from build123d import *

# Parameters (mm, degrees)
F0_W     = 152.4
F0_H     = 1524
F0_W_2   = 114.3
F0_H_2   = 1485.9
F1_DEPTH = 2133.6
F2_W     = 114.3
F2_H     = 19.05
F3_DEPTH = 1485.9
F5_DEPTH = 25.4
F7_DEPTH = 177.8


with BuildPart() as f1:
    # F0 (on Top) → F1 (new body)
    with BuildSketch(Plane.XY):
        Rectangle(F0_W, F0_H)
        Rectangle(F0_W_2, F0_H_2, mode=Mode.SUBTRACT)
    extrude(amount=F1_DEPTH)

    # F2 (on face) → F3 (join)
    with BuildSketch(Plane(origin=(0, -742.95, 0), x_dir=(-1, 0, 0), z_dir=(0, 1, 0))):
        with Locations((0, 2123.313)):
            Rectangle(F2_W, F2_H)
    extrude(amount=F3_DEPTH)

    # F4 (on face) → F5 (cut)
    with BuildSketch(Plane(origin=(-76.2, 0, 0), x_dir=(0, -1, 0), z_dir=(-1, 0, 0))):
        with BuildLine():
            ThreePointArc((30.226, 1625.6), (21.37301, 1646.97301), (0, 1655.826))
            ThreePointArc((0, 1655.826), (-21.37301, 1604.22699), (30.226, 1625.6))
        make_face()
    extrude(amount=-F5_DEPTH, mode=Mode.SUBTRACT)

    # F6 (on face) → F7 (cut)
    with BuildSketch(Plane(origin=(-76.2, 0, 0), x_dir=(0, -1, 0), z_dir=(-1, 0, 0))):
        Polygon((-254, 101.6), (0, 101.6), (254, 101.6), (254, 609.6), (-254, 609.6), align=None)
    extrude(amount=-F7_DEPTH, mode=Mode.SUBTRACT)


solid = f1.part
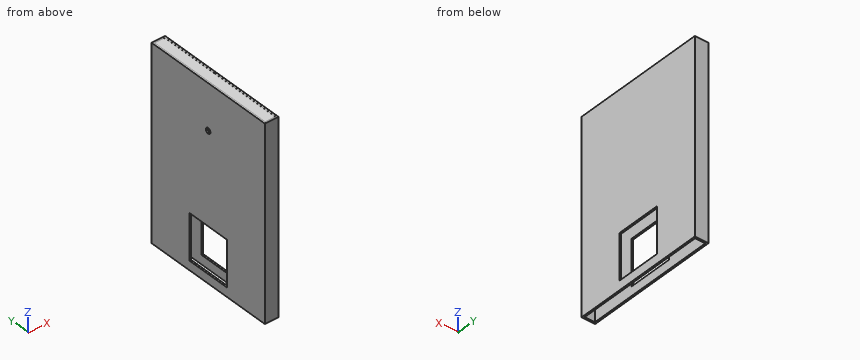
Can you work these out from the model? Positions are in its coordinate system, mm. Give positions to 0.01 mm unless a question says otherwise; leave off trailing zeros. Loops run counter-clockwise (first coordinate to the right, second up) from the corner with the lowest first, then second, coordinate; pieces in that order, holes last. Notation, with made-up numbers: (59, 72.5) -> (80, 72.5) arc R30 cw to (80, 106.5) -> close; hole circle Ø9 at (44.5, 34). An arc over 180 degrees is marked (long way). Return JSON: item names as keys, results as strings.
Q1. I want a section at C-C, the plane z = 295. List the corners of the cut face in (x, y) for me.
Checks:
{"outline": "(-76.2, -762) -> (76.2, -762) -> (76.2, -254) -> (57.15, -254) -> (57.15, -742.95) -> (-57.15, -742.95) -> (-57.15, -254) -> (-76.2, -254) -> close; (-76.2, 254) -> (-57.15, 254) -> (-57.15, 742.95) -> (57.15, 742.95) -> (57.15, 254) -> (76.2, 254) -> (76.2, 762) -> (-76.2, 762) -> close"}
Q2. For pin 1 Ø6 at (x, y) = (-50, 65.5) entering from -Z; pin 2 Ø15 at (x, y) = (-63, -32) entering from -Z; pin 3 Ø6 at (x, y) = (28, -215) entering from +Z, each with a flat end and sliding along its axis, tell me the tip position at first contact or that it passes through.
Checks:
{"pin 1": "stops at z = 2113.79", "pin 2": "stops at z = 0", "pin 3": "stops at z = 2132.84"}
Q3. I want a section at B-B, the plane y = 116.5. List the corners of the cut face in (x, z) for me, then the cut area to 3 significant figures.
Checks:
{"outline": "(-76.2, 0) -> (-57.15, 0) -> (-57.15, 101.6) -> (-76.2, 101.6) -> close; (-76.2, 609.6) -> (-57.15, 609.6) -> (-57.15, 2113.79) -> (57.15, 2113.79) -> (57.15, 609.6) -> (76.2, 609.6) -> (76.2, 2133.6) -> (57.15, 2133.6) -> (57.15, 2132.84) -> (-57.15, 2132.84) -> (-57.15, 2133.6) -> (-76.2, 2133.6) -> close; (57.15, 0) -> (76.2, 0) -> (76.2, 101.6) -> (57.15, 101.6) -> close", "area": "64,100 mm2"}
Q4. I want a section at D-D, the plane x = -24. List the corners of the cut face in (y, z) for me, then the cut area to 3 significant figures.
Checks:
{"outline": "(-762, 0) -> (-742.95, 0) -> (-742.95, 2113.79) -> (742.95, 2113.79) -> (742.95, 0) -> (762, 0) -> (762, 2133.6) -> (742.95, 2133.6) -> (742.95, 2132.84) -> (-742.95, 2132.84) -> (-742.95, 2133.6) -> (-762, 2133.6) -> close", "area": "110,000 mm2"}
Q5. I need wall thicknesses on probe 1 along Y at (x, z) = (-5.5, 932); probe 2 along X at (y, z) = (-309.5, 1115). Which ranges of each line are inside material? Lowest first, please.
Checks:
{"probe 1": "y = -762 to -742.95, 742.95 to 762", "probe 2": "x = -76.2 to -57.15, 57.15 to 76.2"}
Q6. I want a section at A-A, the plane z = 648. List the corners of the cut face in (x, y) for me.
Checks:
{"outline": "(-76.2, -762) -> (76.2, -762) -> (76.2, 762) -> (-76.2, 762) -> close; hole (-57.15, -742.95) -> (57.15, -742.95) -> (57.15, 742.95) -> (-57.15, 742.95) -> close"}
